```python
from build123d import *

# Parameters (mm, degrees)
DRAFT1_ANGLE = 15


with BuildPart() as part:
    # Sketch4 → Revolve1 (revolve)
    with BuildSketch(Plane(origin=(0, 0, 0), x_dir=(1, 0, 0), z_dir=(0, 1, 0))):
        Polygon((0, 101.6), (14, 101.6), (14, 50.8), (8.2, 50.8), (8.2, 25.4), (6.2, 25.4), (6.2, 0), (0, 0), align=None)
    revolve(axis=Axis((0, 0, 0), (0, 0, -1)))

    # Draft1
    draft1_faces = [part.faces().sort_by_distance(p)[0] for p in [
        (-7.968068976, 0, -25.4),
    ]]
    draft(draft1_faces, Plane.ZX, DRAFT1_ANGLE)


solid = part.part
```
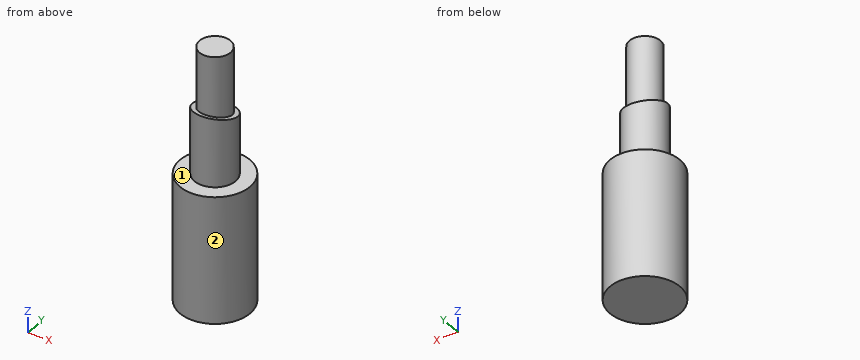
The model under review builds one solid part; all positions refer to its coordinate system, in mm. Face numbers are marked on the shaded views. A direction names the side the tool comes from. Coordinates: 2 decimals unless noted, no trailing zeros. Write each loop counter-clockwise with the first axis right and the second up, starting at its lowest first coordinate (ties: lowest second). Pieces come first, ordered by that corner, then holes. Notation, with made-up numbers: (-4.75, 25) - (14.25, 25) arc R7 ccw to (14.25, 35) - close; hole circle Ø11 at (-36.5, 20.25). An arc over 180 degrees is marked (long way). Answer in a Markdown table with one row per item. Add a question column.
Q1. Consider section B-B on x = 0. Give the boundary of the cut face in (y, z), then the cut area to 3 significant figures.
Q2. To check wall thickness, follow line 1 along Z through (x, y) = (2, -8.25); line 2 along Y through (x, z) = (0, -26.5); line 3 along X through (y, z) = (-1.75, -41.5). State the ranges of each line that lie inside material, in increasing order. Write a range as from..to.
Q3. Consider section D-D on z = -71.5. Give the boundary of the cut face in (x, y).
Q4. For the marked faces 1 and 2, list the 3-axis set-ups (+Z, -Z, +X, -X, +Y, -Y) from which the entire face can be reached by the end or side of a thin tool; tool diameter is ignored.
Q5. Consider section C-C on z = -11. Give the boundary of the cut face in (x, y), then the cut area to 3 significant figures.
Q6. Clearance check with flat-ended pins moving along their axes: pin 1 (8 mm diameter, centred on x = 0.5, z = -13, fed in from +Y); pin 2 (12 mm diameter, centred on x = 5.5, z = -47, fed in from -Y); pin 3 (5 mm diameter, centred on x = -4.5, y = -6, fed in from +Z); pin 4 (5 mm diameter, centred on x = 2, z = -14, fed in from -Y). State where each tip first meets the part, or that it passes through.
Q7. Consider section A-A on y = 0. Give the boundary of the cut face in (x, z), then the cut area to 3 significant figures.
Answers below:
| question | item | result |
|---|---|---|
| 1 | outline | (-14, -101.6) - (14, -101.6) - (14, -50.8) - (8.2, -50.8) - (8.2, -27.6) - (6.2, -27.06) - (6.2, 0) - (-6.2, 0) - (-6.2, -23.74) - (-8.2, -23.2) - (-8.2, -50.8) - (-14, -50.8) - close |
| 1 | area | 2,150 mm² |
| 2 | line 1 | -101.6..-50.8 |
| 2 | line 2 | -8.2..6.2 |
| 2 | line 3 | -8.01..8.01 |
| 3 | outline | circle Ø28 at (0, 0) |
| 4 | face 1 | +Z |
| 4 | face 2 | +Z, -Z |
| 5 | outline | circle Ø12.4 at (0, 0) |
| 5 | area | 121 mm² |
| 6 | pin 1 | y = 6.2 |
| 6 | pin 2 | y = -13.97 |
| 6 | pin 3 | z = 0 |
| 6 | pin 4 | y = -6.2 |
| 7 | outline | (-14, -101.6) - (14, -101.6) - (14, -50.8) - (8.2, -50.8) - (8.2, -25.4) - (6.2, -25.4) - (6.2, 0) - (-6.2, 0) - (-6.2, -25.4) - (-8.2, -25.4) - (-8.2, -50.8) - (-14, -50.8) - close |
| 7 | area | 2,150 mm² |
